Can you work these out from the model? Positions are in its coordinate system, mm. A direction names the side the tool comes from. Round coordinates to 2 decimals unless told otherwise and drop trailing zeros. Loops run counter-clockwise (first coordinate to the right, second up) from the corner with the lowest first, then second, coordinate; pieces in that order, holes last.
(1) I want a section at B-B on x = 16. Write out the boundary of the cut face in (y, z).
(2) Which directions (+Z, -Z, +X, -X, +Y, -Y) give clear straight access to the entire face, cutting with the end or side of a thin tool? Please do faces 5 (the face through (71, -65, 8)), 6 (the face through (81, -55, 8)), 7 (the face through (152, -145, 8)).
(3) I want a section at C-C on y = -60. Write out the boundary of the cut face in (x, z).
(4) If I drill on line 1 along Z through (x, y) = (31, -99.5); line 2 along Y through (x, z) = (140.5, 7.25); line 3 along Y through (x, z) = (72.5, 8.5), over which ranges is the centre line in solid material (lowest first)?
(5) I want a section at D-D on x = 39.5. Write out the boundary of the cut face in (y, z), plus the area to 3 significant figures.
(6) I want a section at A-A on z = 5. Write out the boundary of the cut face in (x, y).
(7) Will these pins go through, and if not, where does the flat tip stop? pin 1 Ø6.5 at (x, z) = (78, 5.5) entering from -Y; pin 2 Ø6.5 at (x, z) = (148, 7.5) entering from +Y; pin 3 Ø8 at (y, z) = (-139.5, 9) entering from +X.
(8) Thinking about a two-plate mould opening in X: for faces 1 (the face through (25, -140, 8)), 2 (the face through (152, -135, 8)), 3 (the face through (137, -140, 8)), 4 (the face through (91, -65, 8)), which applies, released by +X, released by -X, zero draft, split by the parting line, or undercut?
Autodesk Fusion 360 part; units mm, degrees
sketch "Sketch1" plane through (0, 0, 0) normal (0, 0, 1) x (1, 0, 0)
  line L0 (-25, 25) -> (187, 25)
  line L1 (187, 25) -> (187, -155)
  line L2 (187, -155) -> (-25, -155)
  line L3 (-25, -155) -> (-25, 25)
  dimension "d1" = 212
  dimension "d2" = 180
extrude "Extrude1" add sketch "Sketch1" along normal blind 2
sketch "Sketch2" plane through (0, 0, 2) normal (0, 0, 1) x (-1, 0, 0)
  line L0 (25, 155) -> (-187, 155)
  line L1 (-187, 155) -> (-187, -25)
  line L2 (-187, -25) -> (25, -25)
  line L3 (25, -25) -> (25, 155)
  line L4 (25, -25) -> (-187, 155) construction
  line L5 (25, 155) -> (-187, -25) construction
  line L6 (25, 65) -> (-81, 65) construction
  line L7 (-187, 65) -> (-81, 65) construction
  line L8 (-81, 65) -> (-81, -25) construction
  line L9 (-81, 65) -> (-81, 155) construction
  line L10 (25, 155) -> (5, 155) construction
  line L11 (5, 155) -> (5, 135) construction
  line L12 (5, 135) -> (25, 135) construction
  line L13 (25, 135) -> (25, 155) construction
  line L14 (-187, 155) -> (-167, 155) construction
  line L15 (-167, 145) -> (-167, 135)
  line L16 (-167, 135) -> (-187, 135) construction
  line L17 (-187, 135) -> (-187, 155) construction
  line L18 (-187, -25) -> (-167, -25) construction
  line L19 (-167, -25) -> (-167, -5) construction
  line L20 (-167, -5) -> (-187, -5) construction
  line L21 (-187, -5) -> (-187, -25) construction
  line L22 (25, -25) -> (5, -25) construction
  line L23 (5, -25) -> (5, -5) construction
  line L24 (5, -5) -> (25, -5) construction
  line L25 (25, -5) -> (25, -25) construction
  line L26 (-167, 135) -> (-137, 135)
  line L27 (-137, 135) -> (-137, 145)
  line L28 (-137, 145) -> (-167, 145)
  line L29 (-167, 145) -> (-167, 135) construction
  line L30 (5, 135) -> (-25, 135)
  line L31 (-25, 135) -> (-25, 145)
  line L32 (-25, 145) -> (5, 145)
  line L33 (5, 145) -> (5, 135)
  line L34 (-167, 155) -> (-167, 145) construction
  line L35 (-71, 55) -> (-91, 55)
  line L36 (-91, 55) -> (-91, 75)
  line L37 (-91, 75) -> (-71, 75)
  line L38 (-71, 75) -> (-71, 55)
  line L39 (-71, 55) -> (-91, 75) construction
  line L40 (-91, 55) -> (-71, 75) construction
  point P0 (-81, 65)
  dimension "d5" = 20
  dimension "d6" = 20
  dimension "d7" = 20
  dimension "d8" = 20
  dimension "d9" = 20
  dimension "d10" = 20
  dimension "d11" = 20
  dimension "d12" = 20
  dimension "d13" = 30
  dimension "d14" = 10
  dimension "d15" = 30
  dimension "d16" = 10
  dimension "d17" = 20
  dimension "d18" = 20
extrude "Extrude2" add sketch "Sketch2" along normal blind 13 contours L15 L26 L27 L28 | L30 L31 L32 L33 | L35 L36 L37 L38
Filled sheet:
1. outline: (-155, 0) - (25, 0) - (25, 2) - (-135, 2) - (-135, 15) - (-145, 15) - (-145, 2) - (-155, 2) - close
2. face 5: +Z, -X, +Y, -Y
2. face 6: +Z, +X, -X, +Y
2. face 7: +Z, +X, -X, -Y
3. outline: (-25, 0) - (187, 0) - (187, 2) - (91, 2) - (91, 15) - (71, 15) - (71, 2) - (-25, 2) - close
4. line 1: z = 0 to 2
4. line 2: y = -145 to -135
4. line 3: y = -75 to -55
5. outline: (-155, 0) - (25, 0) - (25, 2) - (-155, 2) - close
5. area: 360 mm2
6. outline: (-5, -145) - (25, -145) - (25, -135) - (-5, -135) - close; (71, -75) - (91, -75) - (91, -55) - (71, -55) - close; (137, -145) - (167, -145) - (167, -135) - (137, -135) - close
7. pin 1: stops at y = -75
7. pin 2: stops at y = -135
7. pin 3: stops at x = 167
8. face 1: undercut
8. face 2: zero draft
8. face 3: undercut
8. face 4: released by +X
